from build123d import *

# Parameters (mm, degrees)
SKETCH1_R               = 75
BOSS_EXTRUDE1_DEPTH     = 50
CUT_EXTRUDE1_DEPTH      = 290.39592257
CUT_EXTRUDE1_DEPTH_BACK = 290.39592257
FILLET1_START           = -50
FILLET1_DEPTH           = 100
SKETCH3_R               = 30
CUT_EXTRUDE2_DEPTH      = 303.07614934


with BuildPart() as part:
    # Sketch1 → Boss-Extrude1 (new, symmetric)
    with BuildSketch(Plane.XY):
        with BuildLine():
            Line((-95.945006832, -117.34375), (-36.550478793, 16.25))
            ThreePointArc((-36.550478793, 16.25), (0, 40), (36.550478793, 16.25))
            Line((36.550478793, 16.25), (95.945006832, -117.34375))
            ThreePointArc((95.945006832, -117.34375), (0, -265), (-95.945006832, -117.34375))
        make_face()
        with Locations((0, -160)):
            Circle(SKETCH1_R, mode=Mode.SUBTRACT)
    extrude(amount=BOSS_EXTRUDE1_DEPTH, both=True)

    # Sketch2 → Cut-Extrude1 (cut, two sides: drawn at the far end of the back side and taken through both)
    with BuildSketch(Plane.XY.offset(-CUT_EXTRUDE1_DEPTH_BACK)):
        with BuildLine():
            Line((-35.52920143, -18.375958363), (-82.238577284, -123.4375))
            ThreePointArc((-82.238577284, -123.4375), (0, -70), (82.238577284, -123.4375))
            Line((82.238577284, -123.4375), (35.52920143, -18.375958363))
            ThreePointArc((35.52920143, -18.375958363), (0, -40), (-35.52920143, -18.375958363))
        make_face()
    extrude(amount=CUT_EXTRUDE1_DEPTH + CUT_EXTRUDE1_DEPTH_BACK, mode=Mode.SUBTRACT)

    # Fillet1: read off the stored shape, not the designer's step
    # Fillet1 outline → Fillet1 (add)
    with BuildSketch(Plane.XY.offset(FILLET1_START)):
        with BuildLine():
            ThreePointArc((-42.220939274, -33.427418189), (-35.213916082, -27.719526256), (-26.466655661, -29.991934551))
            ThreePointArc((-26.466655661, -29.991934551), (-31.537347698, -24.604790188), (-35.52920143, -18.375958363))
            Line((-35.52920143, -18.375958363), (-42.220939274, -33.427418189))
        make_face()
        with BuildLine():
            ThreePointArc((35.52920143, -18.375958363), (31.537347698, -24.604790188), (26.466655661, -29.991934551))
            ThreePointArc((26.466655661, -29.991934551), (35.213916082, -27.719526256), (42.220939274, -33.427418189))
            Line((42.220939274, -33.427418189), (35.52920143, -18.375958363))
        make_face()
        with BuildLine():
            ThreePointArc((-43.853361827, -81.406853629), (-55.469552548, -80.058313703), (-57.863577284, -68.61178181))
            Line((-57.863577284, -68.61178181), (-82.238577284, -123.4375))
            ThreePointArc((-82.238577284, -123.4375), (-66.45628703, -99.30764534), (-43.853361827, -81.406853629))
        make_face()
        with BuildLine():
            Line((82.238577284, -123.4375), (57.863577284, -68.61178181))
            ThreePointArc((57.863577284, -68.61178181), (55.469552548, -80.058313703), (43.853361827, -81.406853629))
            ThreePointArc((43.853361827, -81.406853629), (66.45628703, -99.30764534), (82.238577284, -123.4375))
        make_face()
    extrude(amount=FILLET1_DEPTH)

    # Sketch3 → Cut-Extrude2 (cut, through all)
    with BuildSketch(Plane.XY.offset(50)):
        Circle(SKETCH3_R)
    extrude(amount=-CUT_EXTRUDE2_DEPTH, mode=Mode.SUBTRACT)


solid = part.part
The listing builds one solid part. Answer for the finished solid, in the listing's coordinates (mm). A direction names the side the tool comes from. Give positions to 0.01 mm unless a question says otherwise; leave off trailing zeros. Order: outer loops, then holes, each group sorted by start corner. A loop starts at its lowest first (then second) coordinate and runs counter-clockwise, first axis right, second up. Notation, with made-up numbers: (-11, -31.5) - (6, -31.5) arc R19 ccw to (6, -0.5) - close; hole circle Ø11 at (-6, 1.25). An arc over 180 degrees is marked (long way). Answer as CSV lines item,"result".
Q1. Which of the six approach directions +Z, -Z, +X, -X, +Y, -Y give full straight-line access (tool end or side, diameter ignored) to faces 4 (the face through (-49.93, -50.77, -0.7)), 5 (the face through (0, -78, -50))?
Answer key:
face 4,"+Z, -Z"
face 5,"-Z, +X, -X, +Y, -Y"
Q2. Each of these flat-tipped pins is pushed along its axis until it touches: pin 1 Ø3 at (x, z) = (-32.5, 33.5) entering from -Y; pin 2 Ø8 at (y, z) = (-35, -1) entering from -X; pin 3 Ø4 at (x, z) = (68, 17) entering from +Y. Where does it stop, or does it pass through?
Answer key:
pin 1,"stops at y = -260.32"
pin 2,"stops at x = -61.11"
pin 3,"stops at y = -49.99"
Q3. Determine the mould class of faces 1 (the face through (-0.645, 39.995, 0.7)), 2 (the face through (0, -78, 50)), 3 (the face through (-0.6, -70, -0.7)) for opening direction Y: pulls with the +Y half, pulls with the -Y half, needs draft (parallel to the pull), parting line crosses it, or undercut.
Answer key:
face 1,"pulls with the +Y half"
face 2,"needs draft"
face 3,"undercut"
Q4. A cutting plane is placed at B-B, the plane z = -30. Determine the outline of the cut face in (x, y) (3 decimals).
Answer key:
outline,"(-95.945, -117.344) arc R105 ccw (long way) to (95.945, -117.344) - (36.55, 16.25) arc R40 ccw to (-36.55, 16.25) - close; hole circle Ø150 at (0, -160); hole (-57.864, -68.612) arc R10 ccw to (-43.853, -81.407) arc R90 cw to (43.853, -81.407) arc R10 ccw to (57.864, -68.612) - (42.221, -33.427) arc R10 ccw to (26.467, -29.992) arc R40 cw to (-26.467, -29.992) arc R10 ccw to (-42.221, -33.427) - close; hole circle Ø60 at (0, 0)"
Q5. Straight lines are drawn through the part: L1, parallel to Y at x = 1.5, z = -40.5 (1 decimal); L2, parallel to Y at x = -50, z = 34.5; L3, parallel to X at y = -36.5, z = -28. For each, find the intervals that lie inside material, in ascending order.
Answer key:
L1,"y = -265 to -235, -85 to -70, -40 to -30, 30 to 40"
L2,"y = -252.33 to -215.9, -104.1 to -82.59, -50.92 to -14"
L3,"x = -60 to -43.59, -16.36 to 16.36, 43.59 to 60"
Q6. A cutting plane is placed at C-C, the plane x = 1. Determine the outline of the cut face in (y, z).
Answer key:
outline,"(-265, -50) - (-234.99, -50) - (-234.99, 50) - (-265, 50) - close; (-85.01, -50) - (-70.01, -50) - (-70.01, 50) - (-85.01, 50) - close; (-39.99, -50) - (-29.98, -50) - (-29.98, 50) - (-39.99, 50) - close; (29.98, -50) - (39.99, -50) - (39.99, 50) - (29.98, 50) - close"
Q7. A cutting plane is placed at D-D, the plane y = -191.5. Determine the outline of the cut face in (x, z), and give its area (3 significant figures).
Answer key:
outline,"(-100.16, -50) - (-68.06, -50) - (-68.06, 50) - (-100.16, 50) - close; (68.06, -50) - (100.16, -50) - (100.16, 50) - (68.06, 50) - close"
area,"6,420 mm^2"
Q8. A cutting plane is placed at A-A, the plane y = -160. Determine the outline of the cut face in (x, z).
Answer key:
outline,"(-105, -50) - (-75, -50) - (-75, 50) - (-105, 50) - close; (75, -50) - (105, -50) - (105, 50) - (75, 50) - close"
